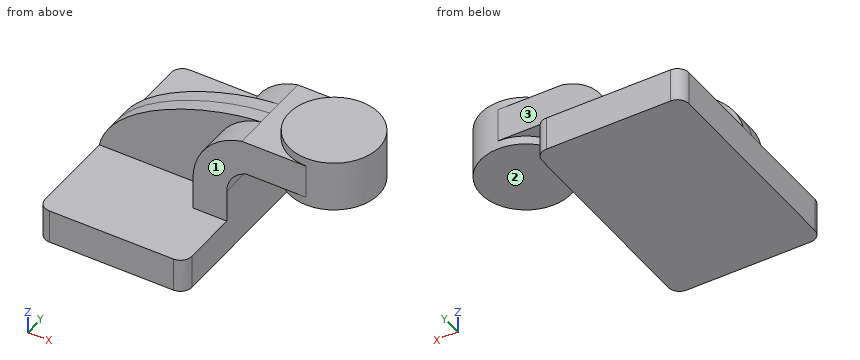
from build123d import *

# Parameters (mm, degrees)
F1_DEPTH = 63.5
F0_W     = 25.5048689127
F0_H     = 19.05
F2_DEPTH = 25.4
F3_DEPTH = 7.9375
F5_R     = 6.35


with BuildPart() as f1:
    # F0 (on Front) → F1 (new body, symmetric)
    with BuildSketch(Plane.XZ):
        Polygon((22.225, 9.525), (-41.275, 9.525), (-41.275, -9.525), (41.275, -9.525), (41.275, 9.525), align=None)
    extrude(amount=F1_DEPTH, both=True)

    # F0 (on Front) → F2 (join, symmetric)
    with BuildSketch(Plane.XZ):
        with BuildLine():
            Line((22.225, 27.7996848035), (22.225, 9.525))
            Line((22.225, 9.525), (41.275, 9.525))
            Line((41.275, 9.525), (41.275, 27.7996848035))
            ThreePointArc((41.275, 27.7996848035), (44.2856320844, 37.1014944732), (52.1756189772, 42.8752))
            Line((52.1756189772, 42.8752), (60.325, 42.8752))
            Line((60.325, 42.8752), (60.325, 61.9252))
            Line((60.325, 61.9252), (49.7200042009, 61.9252))
            ThreePointArc((49.7200042009, 61.9252), (49.7186139898, 61.9248972859), (49.717223791, 61.9245945151))
            ThreePointArc((49.717223791, 61.9245945151), (29.9530761473, 49.7104802695), (22.225, 27.7996848035))
        make_face()
        with Locations((73.0774344563, 52.4002)):
            Rectangle(F0_W, F0_H)
    extrude(amount=F2_DEPTH, both=True)

    # F0 (on Front) → F3 (join, symmetric)
    with BuildSketch(Plane.XZ):
        with BuildLine():
            add(Edge.make_bspline(
                [(-41.275, 9.525), (-35.0649054053, 39.5606108994), (18.1036447727, 59.8387115969), (49.717223791, 61.9245945151)],
                knots=[0, 0, 0, 0, 105.000862147, 105.000862147, 105.000862147, 105.000862147], degree=3))
            Line((-41.275, 9.525), (22.225, 9.525))
            Line((22.225, 9.525), (22.225, 27.7996848035))
            ThreePointArc((22.225, 27.7996848035), (29.9530761473, 49.7104802695), (49.717223791, 61.9245945151))
        make_face()
    extrude(amount=F3_DEPTH, both=True)

    # F0 (on Front) → F4 (revolve)
    with BuildSketch(Plane.XZ):
        Polygon((85.8298689127, 66.675), (85.8298689127, 61.9252), (85.8298689127, 42.8752), (85.8298689127, 38.1), (111.125, 38.1), (111.125, 66.675), align=None)
    revolve(axis=Axis((85.8298689127, 0, 52.3875), (0, 0, 1)))

    # F5
    f5_edges = [f1.edges().sort_by_distance(p)[0] for p in [
        (41.275, 63.5, 0),
        (-41.275, 63.5, 0),
        (-41.275, -63.5, 0),
        (41.275, -63.5, 0),
    ]]
    fillet(f5_edges, radius=F5_R)


solid = f1.part
Model file for the job. Use its own axes, mm. Face numbers are marked on the shaded views. A direction names the side the tool comes from. Give positions to 0.01 mm unless a question says otherwise; leave off trailing zeros. Write each loop counter-clockwise with the first axis right and the second up, starting at its lowest first coordinate (ties: lowest second). Pieces come first, ordered by that corner, then holes. Notation, with made-up numbers: M -18,21.5 L 37,21.5 A33 cw 37,49.5 Z; hole C 6,24.25 d3. An arc over 180 degrees is marked long. One line per item, written item: value. Start each with the question number.
Q1. Drop flat-ended pins along their axis: pin 1 Ø2 at (x, z) = (31.5, 32.5) entering from -Y; pin 2 Ø8.5 at (y, z) = (-18.5, 14.5) entering from -X (3 decimals); pin 3 Ø11 at (x, y) = (60.5, 8.5) entering from +Z (3 decimals); pin 4 Ø15.5 at (x, z) = (0, 28.5) entering from -Y. Give the stop position or say it passes through.
Q2. Probe probe 1 along Y at (x, z) = (37, 35.5); probe 2 along X at (y, z) = (-45, -3.5) (3 decimals); probe 3 along Z at (x, y) = (81, 11) (3 decimals). List the from-to ranges inside material, lowest first. Write a range as [from, to].
Q3. Saw through at B-B, the plane x = 77. Write the cut outline in (y, z) (3 decimals), plus the area to 3 significant figures.
Q4. Saw through at C-C, the plane y = 33. Write the cut outline in (x, z) (3 decimals), plus the area to 3 significant figures.
Q5. Saw through at A-A, the plane z = 1.5. Write the cut outline in (x, y) (3 decimals).
Q6. 3-axis set-ups, long thin cutter, end or side, ignore diameter. For the marked faces 1, 2 and 3: which of +Z, -Z, +X, -X, +Y, -Y reach the whole face in a straight line?
Output values:
1. pin 1: stops at y = -25.4
1. pin 2: stops at x = 22.225
1. pin 3: stops at z = 66.675
1. pin 4: stops at y = -7.94
2. probe 1: y = [-25.4, 25.4]
2. probe 2: x = [-41.275, 41.275]
2. probe 3: z = [38.1, 66.675]
3. outline: M -25.4,42.875 L -23.704,42.875 L -23.704,38.1 L 23.704,38.1 L 23.704,42.875 L 25.4,42.875 L 25.4,61.925 L 23.704,61.925 L 23.704,66.675 L -23.704,66.675 L -23.704,61.925 L -25.4,61.925 Z
3. area: 1,420 mm²
4. outline: M -41.275,-9.525 L 41.275,-9.525 L 41.275,9.525 L -41.275,9.525 Z
4. area: 1,570 mm²
5. outline: M -41.275,-57.15 A6.35 ccw -34.925,-63.5 L 34.925,-63.5 A6.35 ccw 41.275,-57.15 L 41.275,57.15 A6.35 ccw 34.925,63.5 L -34.925,63.5 A6.35 ccw -41.275,57.15 Z
6. face 1: +Z, +X, -X, -Y
6. face 2: -Z, +X, +Y, -Y
6. face 3: +Z, +X, -X, +Y
